Build history of the part. All positions in model axes, mm. Face numbers are marked on the shaded views. A direction names the side the tool comes from. Round coordinates to 2 decimals unless told otherwise and drop trailing zeros. Loops run counter-clockwise (first coordinate to the right, second up) from the corner with the lowest first, then second, coordinate; pieces in that order, holes last. Notation, with made-up numbers: (-8, 67) - (13, 67) arc R21 cw to (13, 72) - close; hole circle Ø3 at (59.25, 56). An arc over 180 degrees is marked (long way). Put each result on its own line as item: value. Start each with the question number.
from build123d import *

# Parameters (mm, degrees)
SKETCH1_W           = 6
SKETCH1_H           = 6
BOSS_EXTRUDE1_DEPTH = 5
CUT_EXTRUDE1_DEPTH  = 10
CUT_EXTRUDE2_DEPTH  = 3


with BuildPart() as part:
    # Sketch1 → Boss-Extrude1 (new body)
    with BuildSketch(Plane(origin=(0, 0, 0), x_dir=(1, 0, 0), z_dir=(0, 1, 0))):
        Rectangle(SKETCH1_W, SKETCH1_H)
    extrude(amount=BOSS_EXTRUDE1_DEPTH)

    # Sketch2 → Cut-Extrude1 (cut)
    with BuildSketch(Plane.ZY.offset(3)):
        Polygon((3, 5), (-3, 5), (0, 2.5), align=None)
    extrude(amount=-CUT_EXTRUDE1_DEPTH, mode=Mode.SUBTRACT)

    # Sketch3 → Cut-Extrude2 (cut)
    with BuildSketch(Plane(origin=(3, 0, 0), x_dir=(0, 0, -1), z_dir=(1, 0, 0))):
        Polygon((-3, 0), (0, 2.5), (-3, 5), align=None)
    extrude(amount=-CUT_EXTRUDE2_DEPTH, mode=Mode.SUBTRACT)


solid = part.part
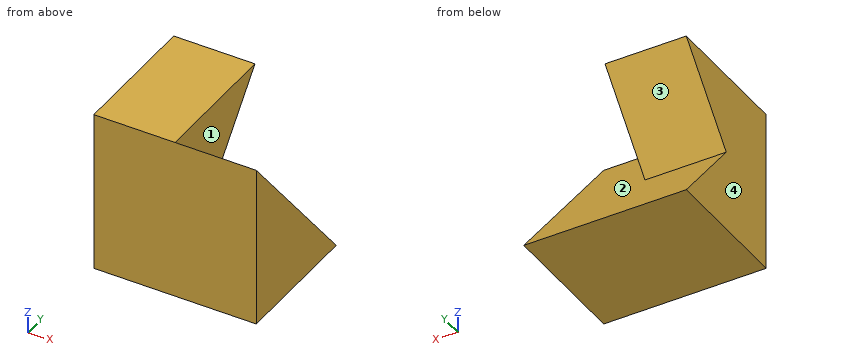
1) Drill centre lines: line 1 (X direction, y = 2.6, z = 2); line 2 (Z direction, x = -0.4, y = 4.1); line 3 (Z direction, x = -2.55, y = 4.65). Where is each one in solid material? Low to high. Write a range as [from, to].
2) Which spindle directions (+Z, -Z, +X, -X, +Y, -Y) get a long thin tool onto all of the face, cutting with end or side? Do the marked faces 1, 2, 3 and 4. Say none if no direction does.
3) Drop a flat-ended pin along its axis: pin 1 Ø1 at (x, z) = (-2, -1.5) entering from +Y. Give the stop position or say it passes through.
4) Slice it at C-C, the plane y = 2.25. Write the cut outline in (x, z), and give its area (3 significant figures).
5) Slice it at A-A, the plane y = 4.5. Write the cut outline in (x, z).
6) Slice it at B-B, the plane x = -1.4. Write the cut outline in (y, z).
7) Slice it at D-D, the plane z = -2.4. Write the cut outline in (x, y), and give its area (3 significant figures).
Taken from the geometry:
1. line 1: x = [-3, 0]
1. line 2: z = [-3, -1.92], [1.92, 3]
1. line 3: z = [-3, -2.58], [2.58, 3]
2. face 1: +Z, +X, +Y
2. face 2: +X, +Y
2. face 3: +X, -X, +Y
2. face 4: +Z, -Z, -X, +Y, -Y
3. pin 1: stops at y = 4.17
4. outline: (-3, -3) - (3, -3) - (3, 0.3) - (0, 0.3) - (0, 3) - (-3, 3) - close
4. area: 27.9 mm2
5. outline: (-3, -3) - (3, -3) - (3, -2.4) - (-3, -2.4) - close; (-3, 2.4) - (0, 2.4) - (0, 3) - (-3, 3) - close
6. outline: (0, -3) - (5, -3) - (2.5, 0) - (5, 3) - (0, 3) - close
7. outline: (-3, 0) - (3, 0) - (3, 4.5) - (-3, 4.5) - close
7. area: 27.0 mm2
